Build history of the part. All positions in model axes, mm. A direction names the side the tool comes from. Round coordinates to 2 decimals unless told otherwise and drop trailing zeros. Write each loop counter-clockwise with the first axis right and the second up, starting at its lowest first coordinate (ties: lowest second). Pieces come first, ordered by that corner, then holes. Notation, with made-up numbers: (-6, 15.25) -> (12, 15.25) arc R35 ccw to (12, 54.25) -> close; hole circle Ø11 at (-13, 5.5). An arc over 180 degrees is marked (long way). Answer in a Markdown table with one row per item.
```python
from build123d import *

# Parameters (mm, degrees)
F0_W     = 47.498
F0_H     = 22.098
F1_DEPTH = 9.652
F3_DEPTH = 7.62
F4_SIZE  = 2.032
F5_W     = 2.032
F5_H     = 7.874
F6_DEPTH = 4.064


with BuildPart() as f1:
    # F0 (on Top) → F1 (new body)
    with BuildSketch(Plane.XY):
        Rectangle(F0_W, F0_H)
    extrude(amount=F1_DEPTH)

    # F2 (on face) → F3 (cut)
    with BuildSketch(Plane.XY.offset(9.652)):
        Polygon((21.717, 9.017), (-21.717, 9.017), (-21.717, 4.28625), (-21.717, -4.28625), (-21.717, -9.017), (21.717, -9.017), align=None)
    extrude(amount=-F3_DEPTH, mode=Mode.SUBTRACT)

    # F4
    f4_edges = [f1.edges().sort_by_distance(p)[0] for p in [
        (0, -11.049, 0),
        (23.749, 0, 0),
        (23.749, -11.049, 4.826),
        (23.749, 11.049, 4.826),
        (-23.749, 0, 0),
        (0, 11.049, 0),
        (-23.749, -11.049, 4.826),
        (-23.749, 11.049, 4.826),
    ]]
    chamfer(f4_edges, length=F4_SIZE)

    # F5 (on face) → F6 (cut)
    with BuildSketch(Plane.XY.offset(9.652)):
        with Locations((-22.733, 0)):
            Rectangle(F5_W, F5_H)
    extrude(amount=-F6_DEPTH, mode=Mode.SUBTRACT)


solid = f1.part
```
Q1. Saw through at A-A on y = -0.75. Write the cut outline in (x, z).
A:
| item | result |
|---|---|
| outline | (-23.75, 2.03) -> (-21.72, 0) -> (21.72, 0) -> (23.75, 2.03) -> (23.75, 9.65) -> (21.72, 9.65) -> (21.72, 2.03) -> (-21.72, 2.03) -> (-21.72, 5.59) -> (-23.75, 5.59) -> close |
Q2. Saw through at D-D on z = 7. Write the cut outline in (x, y), plus the area to 3 significant figures.
A:
| item | result |
|---|---|
| outline | (-23.75, -9.02) -> (-21.72, -11.05) -> (21.72, -11.05) -> (23.75, -9.02) -> (23.75, 9.02) -> (21.72, 11.05) -> (-21.72, 11.05) -> (-23.75, 9.02) -> (-23.75, 3.94) -> (-21.72, 3.94) -> (-21.72, 9.02) -> (21.72, 9.02) -> (21.72, -9.02) -> (-21.72, -9.02) -> (-21.72, -3.94) -> (-23.75, -3.94) -> close |
| area | 242 mm² |
Q3. Wall check: line 1 (X direction, y = -5, z = 8.25); line 2 (Y direction, x = 15.5, z = 7.75); line 3 (Z direction, x = 4.5, y = 1). Give the ranges that are in metal, low to high. Write a range as [from, to].
A:
| item | result |
|---|---|
| line 1 | [-23.75, -21.72], [21.72, 23.75] |
| line 2 | [-11.05, -9.02], [9.02, 11.05] |
| line 3 | [0, 2.03] |
Q4. Drop flat-ended pins along their axis: P1, Ø5, axis at x = 7.5, y = 0.5, coming from the +Z side; P2, Ø3, axis at y = 2, z = 1.5, coming from the -X side; P3, Ø0.6, axis at x = -23, z = 8, coming from the -Y side; P4, Ø1, axis at x = -23, y = 0, coming from the +Z side. Give the stop position or say it passes through.
A:
| item | result |
|---|---|
| P1 | z = 2.03 |
| P2 | x = -23.75 |
| P3 | y = -10.07 |
| P4 | z = 5.59 |
Q5. Saw through at C-C on x = -12. Write the cut outline in (y, z).
A:
| item | result |
|---|---|
| outline | (-11.05, 2.03) -> (-9.02, 0) -> (9.02, 0) -> (11.05, 2.03) -> (11.05, 9.65) -> (9.02, 9.65) -> (9.02, 2.03) -> (-9.02, 2.03) -> (-9.02, 9.65) -> (-11.05, 9.65) -> close |
Q6. Two-plate mould, pull along X, no slides. Class faces 4 (the flat face through (22.493, -9.631, 1.39)), 5 (the flat face through (0, 0, 0)), 6 (the flat face through (-22.331, 9.793, 1.39)), 7 (the flat face through (0, -9.017, 6)): released by +X, released by -X, zero draft, split by the parting line, or undercut.
A:
| item | result |
|---|---|
| face 4 | released by +X |
| face 5 | zero draft |
| face 6 | released by -X |
| face 7 | undercut |
Q7. Saw through at B-B on z = 5. Write the cut outline in (x, y), plus the area to 3 significant figures.
A:
| item | result |
|---|---|
| outline | (-23.75, -9.02) -> (-21.72, -11.05) -> (21.72, -11.05) -> (23.75, -9.02) -> (23.75, 9.02) -> (21.72, 11.05) -> (-21.72, 11.05) -> (-23.75, 9.02) -> close; hole (-21.72, -9.02) -> (21.72, -9.02) -> (21.72, 9.02) -> (-21.72, 9.02) -> close |
| area | 258 mm² |
Q8. Which spindle directions (+Z, -Z, +X, -X, +Y, -Y) get a long thin tool onto all of the face, cutting with end or side? Do faces 1 (the flat face through (0, 9.017, 6)), 2 (the flat face through (0, 11.049, 6)), 3 (the flat face through (-23, 0, 5.588)). Say none if no direction does.
A:
| item | result |
|---|---|
| face 1 | +Z |
| face 2 | +Z, -Z, +X, -X, +Y |
| face 3 | +Z, -X |
